from build123d import *

# Parameters (mm, degrees)
SKETCH6_R                                    = 1.5
BOSS_EXTRUDE4_DEPTH                          = 21.5
SKETCH7_W                                    = 80
SKETCH7_H                                    = 18.040160632
SKETCH7_W_2                                  = 30
SKETCH7_H_2                                  = 6
CUT_EXTRUDE3_DEPTH                           = 18.5
CSK_FOR_M2_COUNTERSUNK_FLAT_HEAD_SCR_2_COUNT = 2
CSK_FOR_M2_COUNTERSUNK_FLAT_HEAD_SCR_2_PITCH = 5
CSK_FOR_M2_COUNTERSUNK_FLAT_HEAD_SCR_3_COUNT = 2
CSK_FOR_M2_COUNTERSUNK_FLAT_HEAD_SCR_3_PITCH = 6
CSK_FOR_M2_COUNTERSUNK_FLAT_HEAD_SCR_4_COUNT = 2
CSK_FOR_M2_COUNTERSUNK_FLAT_HEAD_SCR_4_PITCH = 5
SKETCH90_R                                   = 1.5
CUT_EXTRUDE4_DEPTH                           = 48.575091013


with BuildPart() as part:
    # Sketch6 → Boss-Extrude4 (new, symmetric)
    with BuildSketch(Plane.XY):
        Polygon((-31, 93.5), (-19, 93.5), (-18.392575962, 93.5), (-6.688348482, 99.45725361), (6.688348482, 99.45725361), (18.392575962, 93.5), (19, 93.5), (31, 93.5), (40, 93.5), (40, 97.959320893), (12.976127248, 110.682358229), (6.31198523, 107.009209086), (-6.31198523, 107.009209086), (-12.976127248, 110.682358229), (-40, 97.959320893), (-40, 93.5), align=None)
        with Locations((-13, 105)):
            Circle(SKETCH6_R, mode=Mode.SUBTRACT)
        with Locations(Location((13, 105, 0), (0, 0, 180))):
            Circle(SKETCH6_R, mode=Mode.SUBTRACT)
    extrude(amount=BOSS_EXTRUDE4_DEPTH, both=True)

    # Sketch7 → Cut-Extrude3 (cut, symmetric)
    with BuildSketch(Plane.XY):
        with Locations((0, 105.520080316)):
            Rectangle(SKETCH7_W, SKETCH7_H)
        with Locations((0, 93.5)):
            Rectangle(SKETCH7_W_2, SKETCH7_H_2)
    extrude(amount=CUT_EXTRUDE3_DEPTH, both=True, mode=Mode.SUBTRACT)

    # Sketch89 → CSK for M2 Countersunk Flat Head Screw1 (revolve, cut)
    with BuildSketch(Plane(origin=(-25, 96.5, -3), x_dir=(0, 0, 1), z_dir=(1, 0, 0))):
        Polygon((0, 0), (0, 8.221032743), (1.2, 7.5), (1.2, 1), (2.2, 0), align=None)
    csk_for_m2_countersunk_flat_head_screw1 = revolve(axis=Axis((-25, 102.85, -3), (0, -1, 0)), mode=Mode.SUBTRACT)

    # CSK for M2 Countersunk Flat Head Scr 2: CSK for M2 Countersunk Flat Head Screw1 ×2
    with Locations(*[Vector(0.7999999999999998, 0, 0.6000000000000002) * (i * CSK_FOR_M2_COUNTERSUNK_FLAT_HEAD_SCR_2_PITCH) for i in range(1, CSK_FOR_M2_COUNTERSUNK_FLAT_HEAD_SCR_2_COUNT)]):
        add(csk_for_m2_countersunk_flat_head_screw1, mode=Mode.SUBTRACT)

    # CSK for M2 Countersunk Flat Head Scr 3: CSK for M2 Countersunk Flat Head Screw1 ×2
    with Locations(*[(0, 0, i * CSK_FOR_M2_COUNTERSUNK_FLAT_HEAD_SCR_3_PITCH) for i in range(1, CSK_FOR_M2_COUNTERSUNK_FLAT_HEAD_SCR_3_COUNT)]):
        add(csk_for_m2_countersunk_flat_head_screw1, mode=Mode.SUBTRACT)

    # CSK for M2 Countersunk Flat Head Scr 4: CSK for M2 Countersunk Flat Head Screw1 ×2
    with Locations(*[Vector(-0.8000000000000003, 0, 0.5999999999999996) * (i * CSK_FOR_M2_COUNTERSUNK_FLAT_HEAD_SCR_4_PITCH) for i in range(1, CSK_FOR_M2_COUNTERSUNK_FLAT_HEAD_SCR_4_COUNT)]):
        add(csk_for_m2_countersunk_flat_head_screw1, mode=Mode.SUBTRACT)

    # Mirror1: CSK for M2 Countersunk Flat Head Screw1 across plane
    add(csk_for_m2_countersunk_flat_head_screw1.mirror(Plane(origin=(0, 0, 0), x_dir=(0, 0, 1), z_dir=(1, 0, 0))), mode=Mode.SUBTRACT)

    # Mirror1 copy 1 sketch → Mirror1 copy 1 (revolve, cut)
    with BuildSketch(Plane(origin=(21, 96.5, 0), x_dir=(0, 0, 1), z_dir=(-1, 0, 0))):
        Polygon((0, 0), (0, -8.221032743), (1.2, -7.5), (1.2, -1), (2.2, 0), align=None)
    revolve(axis=Axis((21, 102.85, 0), (0, 1, 0)), mode=Mode.SUBTRACT)

    # Mirror1 copy 2 sketch → Mirror1 copy 2 (revolve, cut)
    with BuildSketch(Plane(origin=(25, 96.5, 3), x_dir=(0, 0, 1), z_dir=(-1, 0, 0))):
        Polygon((0, 0), (0, -8.221032743), (1.2, -7.5), (1.2, -1), (2.2, 0), align=None)
    revolve(axis=Axis((25, 102.85, 3), (0, 1, 0)), mode=Mode.SUBTRACT)

    # Mirror1 copy 3 sketch → Mirror1 copy 3 (revolve, cut)
    with BuildSketch(Plane(origin=(29, 96.5, 0), x_dir=(0, 0, 1), z_dir=(-1, 0, 0))):
        Polygon((0, 0), (0, -8.221032743), (1.2, -7.5), (1.2, -1), (2.2, 0), align=None)
    revolve(axis=Axis((29, 102.85, 0), (0, 1, 0)), mode=Mode.SUBTRACT)

    # Sketch90 → Cut-Extrude4 (cut, through all)
    with BuildSketch(Plane(origin=(0, 96.5, 0), x_dir=(1, 0, 0), z_dir=(0, 1, 0))):
        with Locations(Location((-37, 15.5, 0), (0, 0, 270))):
            Circle(SKETCH90_R)
        with Locations(Location((-37, -15.5, 0), (0, 0, 270))):
            Circle(SKETCH90_R)
        with Locations(Location((37, 15.5, 0), (0, 0, 270))):
            Circle(SKETCH90_R)
        with Locations(Location((37, -15.5, 0), (0, 0, 270))):
            Circle(SKETCH90_R)
    extrude(amount=-CUT_EXTRUDE4_DEPTH, mode=Mode.SUBTRACT)


solid = part.part
Design review of the part built by this model. Coordinates are the model's own, in mm. A direction names the side the tool comes from. Give positions to 0.01 mm unless a question says otherwise; leave off trailing zeros. Loops run counter-clockwise (first coordinate to the right, second up) from the corner with the lowest first, then second, coordinate; pieces in that order, holes last. Notation, with made-up numbers: M 29,50.5 L 62,50.5 A30 cw 62,87.5 Z; hole C 85.25,22 d11. An arc over 180 degrees is marked long. One line per question, with ' | ' between items. Start each with the question number.
1. Add section C-C (x = 29). Write out the cut boundary in (y, z).
2. Add section B-B (z = -15.5). Write out the cut boundary in (x, y).
3. For faces 4 (the face through (-23.83, 94.51, 2.74)), 5 (the face through (0, 99.457, -20)), 6 (the face through (9.69, 108.87, 20.02)), list the 3-axis set-ups (+Z, -Z, +X, -X, +Y, -Y) from which the entire face can be reached by the end or side of a thin tool; tool diameter is ignored.
4. Add section A-A (z = -7). Write out the cut boundary in (x, y).
5. Insertion check: P1, Ø3.5, axis at x = -0.5, z = -20.5, coming from the +Y side; P2, Ø0.9, axis at x = 1, z = 19.5, coming from the -Y side; P3, Ø6, axis at x = -25, z = -0.5, coming from the +Y side. Each pin has a flat end and moves straight along its axis. Give the tip position at first contact, or say it passes through.
6. Add section D-D (z = 0). Give the number of separate pieces and of enclosed holes in the cut face, plus the area to 3 significant figures.
7. To check wall thickness, follow L1, parallel to Z at x = -25, y = 94.45; L2, parallel to X at y = 95.25, z = 15.5; L3, parallel to Z at x = -24, y = 97. State the ranges of each line that lie inside material, in increasing order.
8. The part is to be moulded in two halves that separate along Z. For faces 1 (the face through (36.1, 95, -16.7)), 2 (the face through (-1, 100, 21.5)), 3 (the face through (26.68, 104.23, 20.02)), say which applies: released by +Z, released by -Z, zero draft, split by the parting line, or undercut.
Worked out:
1) outline: M 93.5,-21.5 L 103.14,-21.5 L 103.14,-18.5 L 96.5,-18.5 L 96.5,-2.2 L 95.5,-1.2 L 93.5,-1.2 Z; M 93.5,1.2 L 95.5,1.2 L 96.5,2.2 L 96.5,18.5 L 103.14,18.5 L 103.14,21.5 L 93.5,21.5 Z
2) outline: M -40,93.5 L -38.5,93.5 L -38.5,96.5 L -40,96.5 Z; M -35.5,93.5 L -18.39,93.5 L -15,95.23 L -15,96.5 L -35.5,96.5 Z; M 15,95.23 L 18.39,93.5 L 35.5,93.5 L 35.5,96.5 L 15,96.5 Z; M 38.5,93.5 L 40,93.5 L 40,96.5 L 38.5,96.5 Z
3) face 4: +Y, -Y | face 5: +Z, -Z, -Y | face 6: +Z, -Z, +Y
4) outline: M -40,93.5 L -18.39,93.5 L -15,95.23 L -15,96.5 L -40,96.5 Z; M 15,95.23 L 18.39,93.5 L 40,93.5 L 40,96.5 L 15,96.5 Z
5) P1: stops at y = 107.01 | P2: stops at y = 99.46 | P3: stops at y = 96.5
6) separate pieces: 6 | enclosed holes: 0 | area: 111 mm²
7) L1: z = -21.5 to -4.2, -1.8 to 1.8, 4.2 to 21.5 | L2: x = -40 to -38.5, -35.5 to -15, 15 to 35.5, 38.5 to 40 | L3: z = -21.5 to -18.5, 18.5 to 21.5
8) face 1: undercut | face 2: released by +Z | face 3: zero draft
